For this review, take the finished solid that the model builds, in its own axes (mm). Give positions to 0.01 mm unless a question says otherwise; leave off trailing zeros. Order: outer loops, then holes, each group sorted by start corner. A loop starts at its lowest first (then second) coordinate and runs counter-clockwise, first axis right, second up.
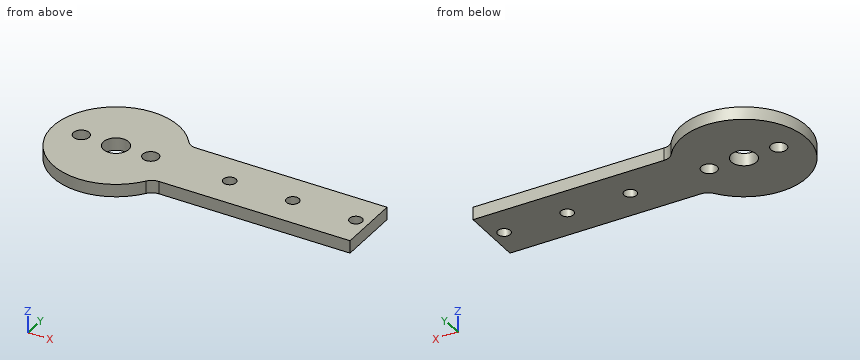
Autodesk Inventor part; units mm, degrees
ref_plane "YZ Plane" through (0, 0, 0) normal (1, 0, 0) x (0, 1, 0)
ref_plane "XZ Plane" through (0, 0, 0) normal (0, 1, 0) x (-1, 0, 0)
ref_plane "XY Plane" through (0, 0, 0) normal (0, 0, 1) x (1, 0, 0)
sketch "スケッチ5" plane through (0, 0, 0) normal (0, 0, 1) x (1, 0, 0)
  circle A0 centre (0, 0) radius 2
  circle A1 centre (0, 0) radius 10
  line L0 (0, 0) -> (40, 0)
  line L1 (40, 0) -> (40, -5)
  line L2 (40, -5) -> (8.6603, -5)
  line L3 (40, 0) -> (40, 5)
  line L4 (40, 5) -> (8.6603, 5)
  circle A2 centre (18, 0) radius 1
  circle A3 centre (28, 0) radius 1
  circle A4 centre (38, 0) radius 1
  circle A5 centre (0, 0) radius 5.5
  circle A6 centre (-5.5, 0) radius 1.25
  circle A7 centre (5.5, 0) radius 1.25
  dimension "d31" = 4
  dimension "d32" = 20
  dimension "d33" = 40
  dimension "d34" = 5
  dimension "d35" = 5
  dimension "d36" = 2
  dimension "d37" = 2
  dimension "d38" = 2
  dimension "d39" = 11
  dimension "d40" = 2.5
  dimension "d41" = 2.5
extrude "押し出し5" add sketch "スケッチ5" along normal blind 2 contours A7 A5 A6 | A1 | A1 L4 L3 L0 A4 A3 A2 | L0 A2 A3 A4 L1 L2 A1
fillet "フィレット2" radius 2 2 edges at (8.6603, 5, 1) (8.6603, -5, 1)
properties part number "cutter_board" material "ABS プラスチック"
1) We need section D-D on x = 26. Give the boundary of the cut face in (y, z), then the cut area to 3 significant figures.
Answer sheet:
outline: (-5, 0) - (5, 0) - (5, 2) - (-5, 2) - close
area: 20.0 mm2
2) To check wall thickness, follow line 1 (Y direction, x = 0, z = 0.55); line 2 (Y direction, x = 38, z = 0.5); line 3 (Y direction, x = 21, z = 1.55). State the ranges of each line that lie inside material, in increasing order.
Answer sheet:
line 1: y = -10 to -2, 2 to 10
line 2: y = -5 to -1, 1 to 5
line 3: y = -5 to 5
3) We need section B-B on z = 0.7. Give the boundary of the cut face in (x, y).
Answer sheet:
outline: (8.12, -5.83) arc R2 cw to (9.75, -5) - (40, -5) - (40, 5) - (9.75, 5) arc R2 cw to (8.12, 5.83) arc R10 ccw (long way) to start; hole circle Ø2.5 at (-5.5, 0); hole circle Ø4 at (0, 0); hole circle Ø2.5 at (5.5, 0); hole circle Ø2 at (18, 0); hole circle Ø2 at (28, 0); hole circle Ø2 at (38, 0)
4) Clearance check with flat-ended pins moving along their axes: pin 1 (1 mm diameter, centred on y = -3.5, z = 2, fed in from -X); pin 2 (0.6 mm diameter, centred on x = 21.5, z = 0.5, fed in from +Y). State where each tip first meets the part, or that it passes through.
Answer sheet:
pin 1: stops at x = -9.54
pin 2: stops at y = 5
5) We need section C-C on x = 0. Give the boundary of the cut face in (y, z).
Answer sheet:
outline: (-10, 0) - (-2, 0) - (-2, 2) - (-10, 2) - close; (2, 0) - (10, 0) - (10, 2) - (2, 2) - close
6) We need section A-A on x = 18. Give the boundary of the cut face in (y, z), then the cut area to 3 significant figures.
Answer sheet:
outline: (-5, 0) - (-1, 0) - (-1, 2) - (-5, 2) - close; (1, 0) - (5, 0) - (5, 2) - (1, 2) - close
area: 16.0 mm2
